For this review, take the finished solid that the model builds, in its own axes (mm). Round coordinates to 2 decimals unless told otherwise and drop trailing zeros. Loops run counter-clockwise (first coordinate to the right, second up) from the corner with the lowest first, then second, coordinate; pieces in that order, holes last. Notation, with made-up numbers: (70, 85.25) -> (114, 85.25) arc R28 ccw to (114, 110.25) -> close; hole circle Ø9 at (86, 50). An arc over 180 degrees is marked (long way). One line per question, with ' | ' between items. Start each with the question number.
1. For pin 1 Ø1.2 at (x, y) = (0, 4) entering from +Z; pin 2 Ø1.5 at (x, z) = (-11.5, 2) entering from +Y; pin 3 Ø1 at (y, z) = (7, 1) entering from -X; pin 4 Ø1 at (y, z) = (13.5, 0.5) entering from -X, all flat-tipped, find the tip position at first contact; note any pin that passes through.
2. Consider section C-C (x = -4). Write out the cut boundary in (y, z), and give its area (3 significant figures).
3. Wall thickness on line 1 along Y through (x, z) = (-10, 1.85); line 2 along Y through (x, z) = (-18, 1.6); line 3 along X through (y, z) = (16, 0.35): over which ranges is each line inside the solid? List them lowest first.
4. Consider section B-B (y = 12). Write out the cut boundary in (x, z).
5. Consider section A-A (z = 1). Write out the cut boundary in (x, y).
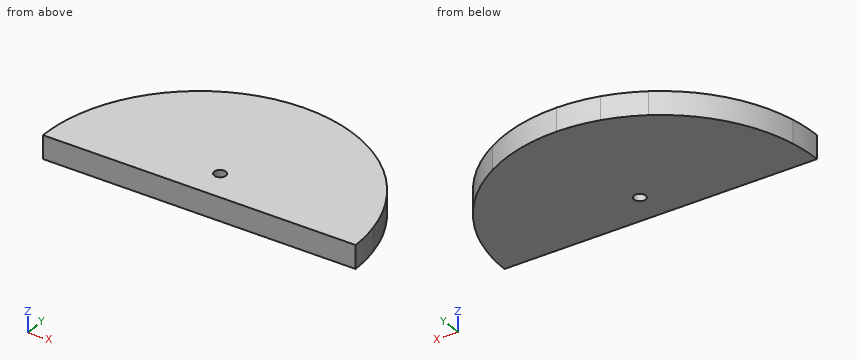
```python
from build123d import *

# Parameters (mm, degrees)
BOSS_EXTRUDE1_DEPTH   = 3
F_1_5MM_DOWEL_HOLE1_D = 1.5


with BuildPart() as part:
    # Sketch1-disc_sketch_2 → Boss-Extrude1 (new body)
    with BuildSketch(Plane.XY):
        with BuildLine():
            ThreePointArc((16.522711642, 4), (16.880256188, 2.01418744), (17, 0))
            Line((17, 0), (20, 0))
            ThreePointArc((20, 0), (19.89872306, 2.01017924), (19.595917942, 4))
            Line((19.595917942, 4), (16.522711642, 4))
        make_face()
        with BuildLine():
            Line((-20, 0), (-17, 0))
            ThreePointArc((-17, 0), (-16.880256188, 2.01418744), (-16.522711642, 4))
            Line((-16.522711642, 4), (-19.595917942, 4))
            ThreePointArc((-19.595917942, 4), (-19.89872306, 2.01017924), (-20, 0))
        make_face()
        with BuildLine():
            ThreePointArc((0, 17), (10.511898021, 13.360389216), (16.522711642, 4))
            Line((16.522711642, 4), (19.595917942, 4))
            ThreePointArc((19.595917942, 4), (16.227710053, 11.690227818), (10, 17.320508076))
            ThreePointArc((10, 17.320508076), (5.176380902, 19.318516526), (0, 20))
            Line((0, 20), (0, 17))
        make_face()
        with BuildLine():
            ThreePointArc((-4.399923767, 16.420739047), (-2.218945268, 16.854562643), (0, 17))
            Line((0, 17), (0, 20))
            ThreePointArc((0, 20), (-2.610523844, 19.828897227), (-5.176380902, 19.318516526))
            Line((-5.176380902, 19.318516526), (-4.399923767, 16.420739047))
        make_face()
        with BuildLine():
            Line((-10, 17.320508076), (-8.5, 14.722431864))
            ThreePointArc((-8.5, 14.722431864), (-6.50561835, 15.705952053), (-4.399923767, 16.420739047))
            Line((-4.399923767, 16.420739047), (-5.176380902, 19.318516526))
            ThreePointArc((-5.176380902, 19.318516526), (-7.653668647, 18.47759065), (-10, 17.320508076))
        make_face()
        with BuildLine():
            Line((-19.595917942, 4), (-16.522711642, 4))
            ThreePointArc((-16.522711642, 4), (-13.611636961, 10.184465585), (-8.5, 14.722431864))
            Line((-8.5, 14.722431864), (-10, 17.320508076))
            ThreePointArc((-10, 17.320508076), (-16.227710053, 11.690227818), (-19.595917942, 4))
        make_face()
        with BuildLine():
            Line((-17, 0), (-3, 0))
            ThreePointArc((-3, 0), (-2.598076211, 1.5), (-1.5, 2.598076211))
            Line((-1.5, 2.598076211), (-2.309401077, 4))
            Line((-2.309401077, 4), (-16.522711642, 4))
            ThreePointArc((-16.522711642, 4), (-16.880256188, 2.01418744), (-17, 0))
        make_face()
        with BuildLine():
            ThreePointArc((0, 3), (2.121320344, 2.121320344), (3, 0))
            Line((3, 0), (17, 0))
            ThreePointArc((17, 0), (16.880256188, 2.01418744), (16.522711642, 4))
            Line((16.522711642, 4), (0, 4))
            Line((0, 4), (0, 3))
        make_face()
        with BuildLine():
            Line((0, 17), (0, 4))
            Line((0, 4), (16.522711642, 4))
            ThreePointArc((16.522711642, 4), (10.511898021, 13.360389216), (0, 17))
        make_face()
        with BuildLine():
            Line((-1.07179677, 4), (0, 4))
            Line((0, 4), (0, 17))
            ThreePointArc((0, 17), (-2.218945268, 16.854562643), (-4.399923767, 16.420739047))
            Line((-4.399923767, 16.420739047), (-1.07179677, 4))
        make_face()
        with BuildLine():
            Line((-8.5, 14.722431864), (-2.309401077, 4))
            Line((-2.309401077, 4), (-1.07179677, 4))
            Line((-1.07179677, 4), (-4.399923767, 16.420739047))
            ThreePointArc((-4.399923767, 16.420739047), (-6.50561835, 15.705952053), (-8.5, 14.722431864))
        make_face()
        with BuildLine():
            Line((-16.522711642, 4), (-2.309401077, 4))
            Line((-2.309401077, 4), (-8.5, 14.722431864))
            ThreePointArc((-8.5, 14.722431864), (-13.611636961, 10.184465585), (-16.522711642, 4))
        make_face()
        with BuildLine():
            Line((-2.309401077, 4), (-1.5, 2.598076211))
            ThreePointArc((-1.5, 2.598076211), (-1.148050297, 2.771638598), (-0.776457135, 2.897777479))
            Line((-0.776457135, 2.897777479), (-1.07179677, 4))
            Line((-1.07179677, 4), (-2.309401077, 4))
        make_face()
        with BuildLine():
            ThreePointArc((-0.776457135, 2.897777479), (-0.391578577, 2.974334584), (0, 3))
            Line((0, 3), (0, 4))
            Line((0, 4), (-1.07179677, 4))
            Line((-1.07179677, 4), (-0.776457135, 2.897777479))
        make_face()
        with BuildLine():
            Line((-3, 0), (0, 0))
            Line((0, 0), (-1.5, 2.598076211))
            ThreePointArc((-1.5, 2.598076211), (-2.598076211, 1.5), (-3, 0))
        make_face()
        with BuildLine():
            Line((-1.5, 2.598076211), (0, 0))
            Line((0, 0), (-0.776457135, 2.897777479))
            ThreePointArc((-0.776457135, 2.897777479), (-1.148050297, 2.771638598), (-1.5, 2.598076211))
        make_face()
        with BuildLine():
            Line((-0.776457135, 2.897777479), (0, 0))
            Line((0, 0), (0, 3))
            ThreePointArc((0, 3), (-0.391578577, 2.974334584), (-0.776457135, 2.897777479))
        make_face()
        with BuildLine():
            Line((0, 3), (0, 0))
            Line((0, 0), (3, 0))
            ThreePointArc((3, 0), (2.121320344, 2.121320344), (0, 3))
        make_face()
    extrude(amount=BOSS_EXTRUDE1_DEPTH)

    # 1.5mm Dowel Hole1 (through all)
    with Locations(Plane.XY.offset(3)):
        with Locations((0, 4)):
            Hole(F_1_5MM_DOWEL_HOLE1_D / 2)


solid = part.part
```
Answer block:
1) pin 1: passes through | pin 2: stops at y = 16.87 | pin 3: stops at x = -18.91 | pin 4: stops at x = -15.2
2) outline: (0, 0) -> (19.6, 0) -> (19.6, 3) -> (0, 3) -> close | area: 58.8 mm2
3) line 1: y = 0 to 17.32 | line 2: y = 0 to 8.72 | line 3: x = -12 to 12
4) outline: (-16, 0) -> (16, 0) -> (16, 3) -> (-16, 3) -> close
5) outline: (-20, 0) -> (20, 0) arc R20 ccw to start; hole circle Ø1.5 at (0, 4)
